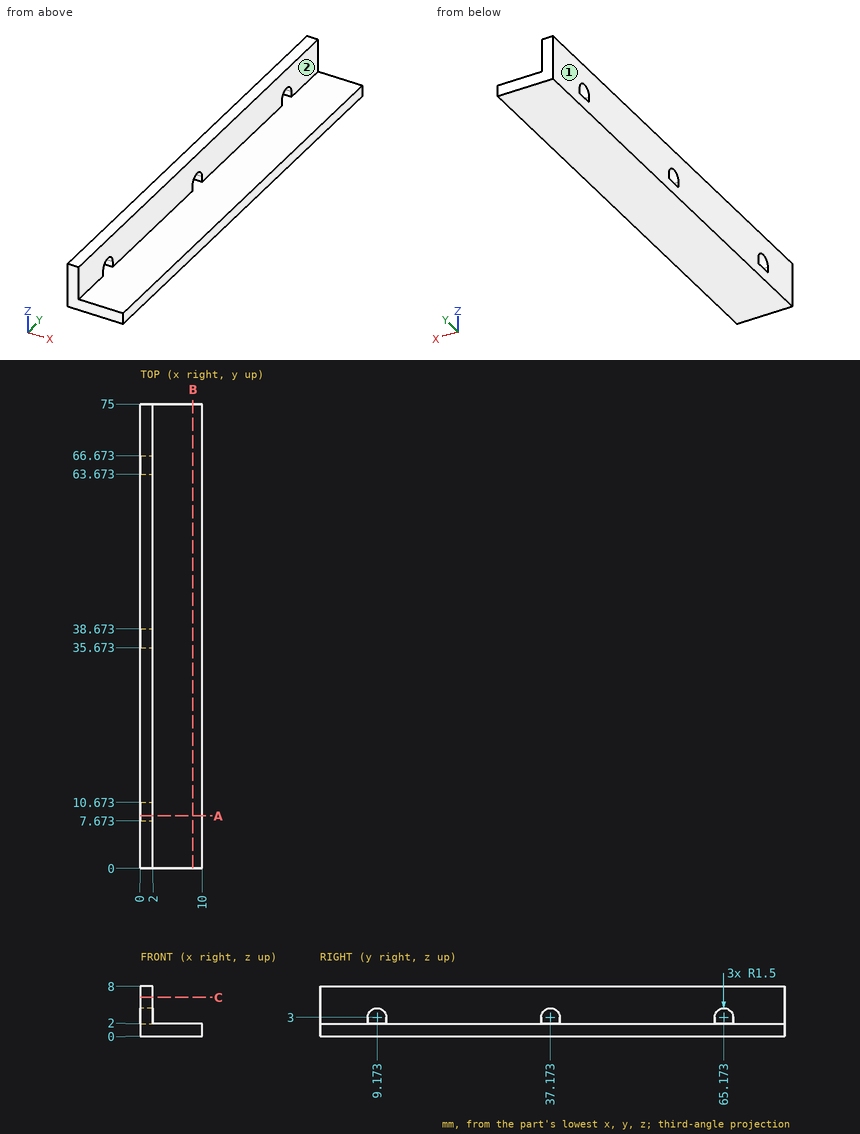
Geometry: see drawing. Coordinates: mm, zero at the bounding-box minimum. A direction names the side the tool comes from. Coordinates: 2 decimals unless noted, no trailing zeros. Write each loop counter-clockwise with the first axis right and the second up, starting at its lowest first coordinate (ties: lowest second). Pieces come first, ordered by that corner, then holes. Notation, with made-up numbers: M -29,-39.5 L -19,-39.5 A23 cw -19,-28.5 Z; hole C -28.75,7 d8. An arc over 180 degrees is marked long. Use CSV: the item, a comma, the result in double quotes. Start each with the question number.
1. Cut plane B-B on x = 8.5. Return the cut outline in (y, z).
2. Ray query, probe 1 along Z at (x, y) = (4.75, 10.5). Return the intervals inside material, ascending.
3. Reachability of the marked faces 1 and 2 from +Z, -Z, +X, -X, +Y, -Y: full face, straight path, thin tool, end or side. Return the list, or none.
4. Cut plane C-C on z = 6.25. Return the cut outline in (x, y), plus the area to 3 significant figures.
5. Cut plane A-A on y = 8.5. Return the cut outline in (x, z).
6. First-contact query: P1, Ø3, axis at y = 34, z = 5.5, coming from the +X side. Flat tip, straight axial feed; report the tip coordinate or a pass-through.
Entries:
1,outline,"M 0,0 L 75,0 L 75,2 L 0,2 Z"
2,probe 1,"0 to 2"
3,face 1,"+Z, -Z, -X, +Y, -Y"
3,face 2,"+Z, +X, +Y, -Y"
4,outline,"M 0,0 L 2,0 L 2,75 L 0,75 Z"
4,area,"150 mm²"
5,outline,"M 0,0 L 10,0 L 10,2 L 0,2 Z; M 0,4.34 L 2,4.34 L 2,8 L 0,8 Z"
6,P1,"x = 2"
